Autodesk Inventor part; units mm, degrees
ref_plane "YZ Plane" through (0, 0, 0) normal (1, 0, 0) x (0, 1, 0)
ref_plane "XZ Plane" through (0, 0, 0) normal (0, 1, 0) x (-1, 0, 0)
ref_plane "XY Plane" through (0, 0, 0) normal (0, 0, 1) x (1, 0, 0)
sketch "Sketch1" plane through (0, 0, 0) normal (1, 0, 0) x (0, 1, 0)
  line L0 (0, 0) -> (50.8, 0)
  line L1 (50.8, 0) -> (50.8, -76.2)
  line L2 (50.8, -76.2) -> (0, -76.2)
  line L3 (0, -76.2) -> (0, 0)
  line L4 (50.8, -6.35) -> (6.35, -6.35)
  line L5 (6.35, -6.35) -> (6.35, -69.85)
  line L6 (6.35, -69.85) -> (50.8, -69.85)
  line L7 (50.8, -69.85) -> (50.8, -6.35)
  dimension "d0" = 50.8
  dimension "d1" = 76.2
  dimension "d2" = 6.35
  dimension "d3" = 6.35
  dimension "d4" = 6.35
extrude "Extrusion1" add sketch "Sketch1" along normal blind 25.4 contours L0 L1 L4 L5 L6 L2 L3
sketch "Sketch2" plane through (0, 0, 0) normal (0, 0, 1) x (1, 0, 0)
  line L0 (0, 50.8) -> (0, 0)
  line L1 (0, 0) -> (25.4, 0)
  line L2 (25.4, 50.8) -> (25.4, 0)
  line L3 (0, 50.8) -> (25.4, 50.8)
  point P0 (12.7, 38.1)
  dimension "d7" = 12.7
  dimension "d8" = 12.7
hole "Hole1" at (12.7, 38.1, 0) direction (0, 0, -1) diameter 6.35 end through all
properties part number "StressProngs"
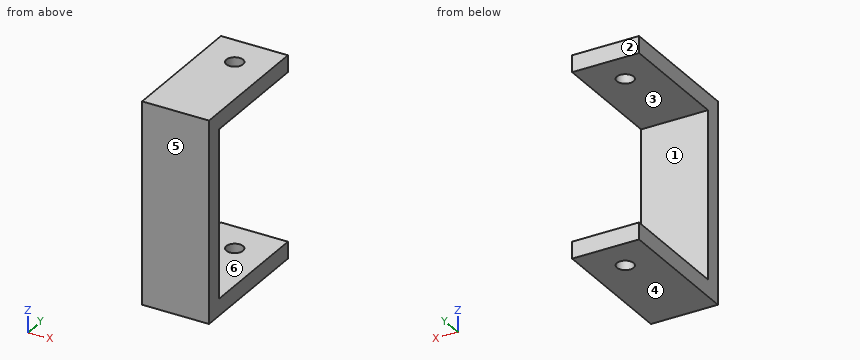
Verification items for the finished model (mm, model axes). Face numbers are marked on the shaded views. A direction names the side the tool comes from. Give positions to 0.01 mm unless a question says otherwise; leave off trailing zeros. Write each loop counter-clockwise with the first axis right and the second up, starting at its lowest first coordinate (ties: lowest second). Pieces come first, ordered by that corner, then holes. Notation, with made-up numbers: (24, 75.25) - (43, 75.25) arc R22 ccw to (43, 97.25) - close; hole circle Ø7 at (-2.5, 73). An arc over 180 degrees is marked (long way). Answer as CSV lines item,"result". Start each with the question number.
1. Depth check by flat-ended pin: pin 1 (1 mm diameter, centred on x = 16.5, z = -62.5, fed in from +Y); pin 2 (5 mm diameter, centred on x = 12.7, y = 38.1, fed in from -Z). Enter the tip coordinate at first touch or a pass-through.
2. Sectioned sample at B-B (y = 38.1). Record the boundary of the cut face in (x, z) (3 decimals).
3. Thickness scan on line 1 (Z direction, x = 9, y = 48.5); line 2 (Y direction, x = 12.7, z = -74.5) (3 decimals); line 3 (X direction, y = 38.1, z = -72.5) (3 decimals). Record the ranges inside material, lowest first.
4. Sectioned sample at A-A (x = 12.7). Record the boundary of the cut face in (y, z) (3 decimals), then the cut area to 3 significant figures.
5. Draft check along Z on the marked faces 1, 2, 3 and 4. Enter one of: pulls with the +Z half, pulls with the -Z half, needs draft (parallel to the pull), parting line crosses it, or undercut.
6. Sectioned sample at C-C (y = 17.5). Record the boundary of the cut face in (x, z), then the cut area to 3 significant figures.
7. Sectioned sample at D-D (z = -5.5). Record the boundary of the cut face in (x, y) (3 decimals).
8. Set-up check for the marked faces 5 and 6: record each of +Z, -Z, +X, -X, +Y, -Y from which the full face is reachable in a straight line by a thin tool's end or side.
Derived:
1,pin 1,"y = 6.35"
1,pin 2,"through"
2,outline,"(0, -76.2) - (9.525, -76.2) - (9.525, -69.85) - (0, -69.85) - close; (0, -6.35) - (9.525, -6.35) - (9.525, 0) - (0, 0) - close; (15.875, -76.2) - (25.4, -76.2) - (25.4, -69.85) - (15.875, -69.85) - close; (15.875, -6.35) - (25.4, -6.35) - (25.4, 0) - (15.875, 0) - close"
3,line 1,"-76.2 to -69.85, -6.35 to 0"
3,line 2,"0 to 34.925, 41.275 to 50.8"
3,line 3,"0 to 9.525, 15.875 to 25.4"
4,outline,"(0, -76.2) - (34.925, -76.2) - (34.925, -69.85) - (6.35, -69.85) - (6.35, -6.35) - (34.925, -6.35) - (34.925, 0) - (0, 0) - close; (41.275, -76.2) - (50.8, -76.2) - (50.8, -69.85) - (41.275, -69.85) - close; (41.275, -6.35) - (50.8, -6.35) - (50.8, 0) - (41.275, 0) - close"
4,area,"968 mm²"
5,face 1,"undercut"
5,face 2,"needs draft"
5,face 3,"undercut"
5,face 4,"pulls with the -Z half"
6,outline,"(0, -76.2) - (25.4, -76.2) - (25.4, -69.85) - (0, -69.85) - close; (0, -6.35) - (25.4, -6.35) - (25.4, 0) - (0, 0) - close"
6,area,"323 mm²"
7,outline,"(0, 0) - (25.4, 0) - (25.4, 50.8) - (0, 50.8) - close; hole circle Ø6.35 at (12.7, 38.1)"
8,face 5,"+Z, -Z, +X, -X, -Y"
8,face 6,"+X, -X, +Y"
